Input: part model. Units: mm. Frame: model coordinates. Round coordinates to 2 decimals unless told otherwise and drop trailing zeros. Loops run counter-clockwise (first coordinate to the right, second up) from the corner with the lowest first, then second, coordinate; pieces in that order, holes last. Notation, with made-up numbers: (13, 10) - (46, 10) arc R28 ccw to (46, 41) - close; hole circle Ø2 at (54.5, 84.5). An arc over 180 degrees is marked (long way). Write each question's results on one line, items separated by ' | '.
from build123d import *

# Parameters (mm, degrees)
IZIM1_W                     = 360
IZIM1_H                     = 120
IZIM1_W_2                   = 302.16
IZIM1_H_2                   = 8
Y_KSEKLIK_EKSTR_ZYON1_DEPTH = 8
IZIM4_W                     = 16
IZIM4_H                     = 100
KES_EKSTR_ZYON3_DEPTH       = 10
IZIM5_W                     = 35
IZIM5_H                     = 8
IZIM5_W_2                   = 10.030547984
IZIM5_W_3                   = 10
KES_EKSTR_ZYON4_DEPTH       = 8


with BuildPart() as part:
    # Çizim1 → Yükseklik-Ekstrüzyon1 (new body)
    # profile 1 of 3: a face of its own
    with BuildSketch(Plane.XY):
        with Locations((-70.427590571, -6.826190476)):
            Rectangle(IZIM1_W, IZIM1_H)
        with Locations((-70.427590571, 1.173809524)):
            Rectangle(IZIM1_W_2, IZIM1_H_2, mode=Mode.SUBTRACT)
        with Locations((-70.427590571, -14.826190476)):
            Rectangle(IZIM1_W_2, IZIM1_H_2, mode=Mode.SUBTRACT)
    # profile 2 of 3: a face of its own
    with BuildSketch(Plane.XY):
        with Locations((-70.427590571, -14.826190476)):
            Rectangle(IZIM1_W_2, IZIM1_H_2)
    # profile 3 of 3: a face of its own
    with BuildSketch(Plane.XY):
        with Locations((-70.427590571, 1.173809524)):
            Rectangle(IZIM1_W_2, IZIM1_H_2)
    extrude(amount=Y_KSEKLIK_EKSTR_ZYON1_DEPTH)

    # Çizim4 → Kes-Ekstrüzyon3 (cut)
    with BuildSketch(Plane(origin=(0, 0, 0), x_dir=(-1, 0, 0), z_dir=(0, 0, -1))):
        with Locations((232.427590571, -6.826190476)):
            Rectangle(IZIM4_W, IZIM4_H)
        with Locations((-91.572409429, -6.826190476)):
            Rectangle(IZIM4_W, IZIM4_H)
    extrude(amount=-KES_EKSTR_ZYON3_DEPTH, mode=Mode.SUBTRACT)

    # Çizim5 → Kes-Ekstrüzyon4 (cut)
    with BuildSketch(Plane.XY.offset(8)):
        with Locations((-145.442864563, 1.173809524)):
            Rectangle(IZIM5_W, IZIM5_H)
        with Locations((-145.412316579, -14.826190476)):
            Rectangle(IZIM5_W, IZIM5_H)
        with Locations((-182.927590571, -14.826190476)):
            Rectangle(IZIM5_W_2, IZIM5_H)
        with Locations((-182.942864563, 1.173809524)):
            Rectangle(IZIM5_W_3, IZIM5_H)
        with Locations((-95.412316579, -14.826190476)):
            Rectangle(IZIM5_W, IZIM5_H)
        with Locations((-95.442864563, 1.173809524)):
            Rectangle(IZIM5_W, IZIM5_H)
        with Locations((-45.412316579, -14.826190476)):
            Rectangle(IZIM5_W, IZIM5_H)
        with Locations((-45.442864563, 1.173809524)):
            Rectangle(IZIM5_W, IZIM5_H)
        with Locations((4.587683421, -14.826190476)):
            Rectangle(IZIM5_W, IZIM5_H)
        with Locations((4.557135437, 1.173809524)):
            Rectangle(IZIM5_W, IZIM5_H)
        with Locations((42.087683421, -14.826190476)):
            Rectangle(IZIM5_W_3, IZIM5_H)
        with Locations((42.072409429, 1.173809524)):
            Rectangle(IZIM5_W_2, IZIM5_H)
    extrude(amount=-KES_EKSTR_ZYON4_DEPTH, mode=Mode.SUBTRACT)


solid = part.part
1. Section query B-B, the plane x = -184. Output: boundary loops of the cut face in (y, z).
Answer:
outline: (-66.83, 0) - (-18.83, 0) - (-18.83, 8) - (-66.83, 8) - close; (-10.83, 0) - (-2.83, 0) - (-2.83, 8) - (-10.83, 8) - close; (5.17, 0) - (53.17, 0) - (53.17, 8) - (5.17, 8) - close
2. Section query A-A, the plane y = -33. Output: boundary loops of the cut face in (x, z), plus the area to 3 significant figures.
Answer:
outline: (-250.43, 0) - (-240.43, 0) - (-240.43, 8) - (-250.43, 8) - close; (-224.43, 0) - (83.57, 0) - (83.57, 8) - (-224.43, 8) - close; (99.57, 0) - (109.57, 0) - (109.57, 8) - (99.57, 8) - close | area: 2,620 mm^2
3. Section query C-C, the plane z = 6.25. Count the separate pieces of the cut face and the enclosed holes in it, plus the area to 3 significant figures.
Answer:
separate pieces: 1 | enclosed holes: 14 | area: 37,400 mm^2
4. Mould query, pull axis Y, two halves, no side actions, for faces 1 (the flat face through (99.572, -8, 4)), 2 (the flat face through (109.572, -8, 4)). Classes: pulls with the +Y half, pulls with the -Y half, needs draft (parallel to the pull), parting line crosses it, or undercut.
Answer:
face 1: undercut | face 2: needs draft
5. Line query: line 1 (Y direction, x = 20, z = 7); line 2 (X direction, y = -49, z = 5.25). Output: solid intervals per line, ascending. Write a range as [from, to].
Answer:
line 1: [-66.83, -18.83], [-10.83, -2.83], [5.17, 53.17] | line 2: [-250.43, -240.43], [-224.43, 83.57], [99.57, 109.57]
